The model under review builds one solid part; all positions refer to its coordinate system, in mm. Face numbers are marked on the shaded views. Round coordinates to 2 decimals unless told otherwise and drop trailing zeros. Loops run counter-clockwise (first coordinate to the right, second up) from the corner with the lowest first, then second, coordinate; pieces in that order, holes last. Notation, with made-up numbers: (53, 23.25) -> (105, 23.25) arc R19 cw to (105, 46.25) -> close; hole circle Ø2 at (54, 82.25). An arc over 180 degrees is marked (long way). Use a Markdown table: item, result. Add a question column.
1) Consider section B-B on y = 2. Give the boundary of the cut face in (x, z), plus the area to 3 significant figures.
2) Wall thickness on probe 1 along X at (y, z) = (3, -20.5); probe 2 along Z at (x, y) = (5.75, 3.25); probe 3 along Z at (x, y) = (6.75, 1.75): over which ranges is each line inside the solid? List them lowest first.
3) Consider section D-D on x = 6.75. Give the boundary of the cut face in (y, z), plus the area to 3 significant figures.
4) Consider section C-C on x = 16.25. Give the boundary of the cut face in (y, z), plus the area to 3 significant figures.
5) Insertion check: pin 1 (1 mm diameter, centred on y = 1, z = -19.5, fed in from -X); pin 2 (12 mm diameter, centred on x = 2.5, z = -4, fed in from -Y). Each pin has a flat end and moves straight along its axis. Give the tip position at first contact, or say it passes through.
6) Consider section A-A on z = -14. Give the boundary of the cut face in (x, y), plus the area to 3 significant figures.
7) Mouldability with a two-part tool opening along Z and no side actions: class the marked faces 1, 2 and 3 as released by +Z, released by -Z, zero draft, split by the parting line, or undercut.
from build123d import *

# Parameters (mm, degrees)
BOSS_EXTRUDE1_DEPTH = 6.35


with BuildPart() as part:
    # Sketch1 → Boss-Extrude1 (new body)
    with BuildSketch(Plane(origin=(0, 0, 0), x_dir=(1, 0, 0), z_dir=(0, 1, 0))):
        with BuildLine():
            Line((0, 0), (25.4, 0))
            Line((25.4, 0), (25.4, 14.863926823))
            ThreePointArc((25.4, 14.863926823), (25.182699479, 18.179292106), (24.534515988, 21.437930569))
            Line((24.534515988, 21.437930569), (24.413899438, 21.88807766))
            ThreePointArc((24.413899438, 21.88807766), (23.230447839, 23.430381811), (21.303047465, 23.684128884))
            Line((21.303047465, 23.684128884), (20.977173177, 23.596811132))
            ThreePointArc((20.977173177, 23.596811132), (19.434869026, 22.413359533), (19.181121952, 20.485959159))
            Line((19.181121952, 20.485959159), (20.167222514, 16.80578176))
            Line((20.167222514, 16.80578176), (8.636, 13.716))
            Line((8.636, 13.716), (7.490177398, 17.992268167))
            ThreePointArc((7.490177398, 17.992268167), (3.312695208, 20.783572527), (0, 17.006167605))
            Line((0, 17.006167605), (0, 0))
        make_face()
    extrude(amount=BOSS_EXTRUDE1_DEPTH)


solid = part.part
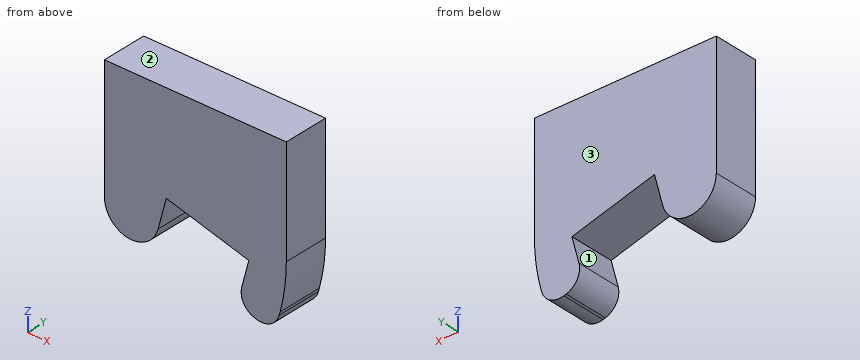
Result set:
| question | item | result |
|---|---|---|
| 1 | outline | (0, -17.01) arc R3.81 ccw to (7.49, -17.99) -> (8.64, -13.72) -> (20.17, -16.81) -> (19.18, -20.49) arc R2.54 ccw to (20.98, -23.6) -> (21.3, -23.68) arc R2.54 ccw to (24.41, -21.89) -> (24.53, -21.44) arc R25.4 ccw to (25.4, -14.86) -> (25.4, 0) -> (0, 0) -> close |
| 1 | area | 467 mm2 |
| 2 | probe 1 | 2.29 to 5.33, 19.18 to 24.77 |
| 2 | probe 2 | -20.29 to 0 |
| 2 | probe 3 | -19.43 to 0 |
| 3 | outline | (0, -19.43) -> (6.35, -19.43) -> (6.35, 0) -> (0, 0) -> close |
| 3 | area | 123 mm2 |
| 4 | outline | (0, -15.76) -> (6.35, -15.76) -> (6.35, 0) -> (0, 0) -> close |
| 4 | area | 100 mm2 |
| 5 | pin 1 | x = 0.56 |
| 5 | pin 2 | y = 0 |
| 6 | outline | (0, 0) -> (8.56, 0) -> (8.56, 6.35) -> (0, 6.35) -> close; (9.7, 0) -> (25.4, 0) -> (25.4, 6.35) -> (9.7, 6.35) -> close |
| 6 | area | 154 mm2 |
| 7 | face 1 | undercut |
| 7 | face 2 | released by +Z |
| 7 | face 3 | zero draft |
